Geometry check sheet. Reference: the model listing, model coordinates, mm. Face numbers are marked on the shaded views. A direction names the side the tool comes from. Coordinates: 2 decimals unless noted, no trailing zeros. Order: outer loops, then holes, each group sorted by start corner. A loop starts at its lowest first (then second) coordinate and runs counter-clockwise, first axis right, second up. Notation, with made-up numbers: M 88,-29.75 L 124,-29.75 A25 cw 124,-12.75 Z; hole C -5.75,82 d10. An arc over 180 degrees is marked long. Use CSV: the item, a comma, the result in double quotes. Start each with the question number.
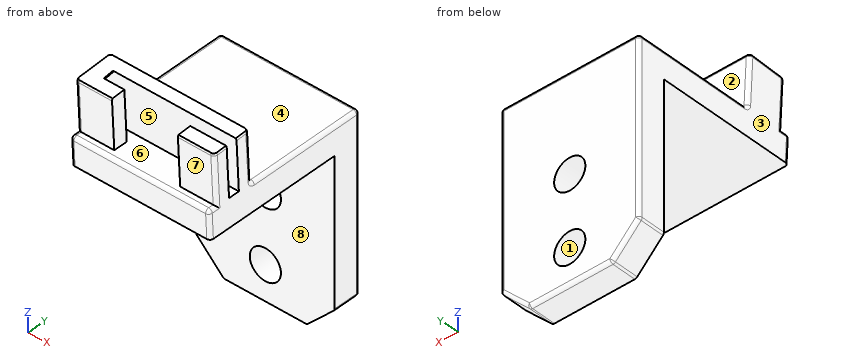
```python
from build123d import *

# Parameters (mm, degrees)
SKETCH1_W                       = 25.4
SKETCH1_H                       = 31.75
SKETCH1_R                       = 2.8575
BOSS_EXTRUDE1_DEPTH             = 5.08
BOSS_EXTRUDE2_REACH             = 22.955
BOSS_EXTRUDE2_DIRECTION_2_REACH = 22.955
CUT_EXTRUDE3_REACH              = 56.752
BOSS_EXTRUDE3_DEPTH             = 2
BOSS_EXTRUDE3_DRAFT             = -3
CHAMFER1_SIZE                   = 5.08
FILLET1_R                       = 0.635
SKETCH8_W                       = 25.4
SKETCH8_H                       = 6.35
CUT_EXTRUDE4_DEPTH              = 41.010145227


with BuildPart() as part:
    # Sketch1 → Boss-Extrude1 (new body)
    with BuildSketch(Plane(origin=(0, 0, 0), x_dir=(1, 0, 0), z_dir=(0, 1, 0))):
        Rectangle(SKETCH1_W, SKETCH1_H)
        with Locations(Location((0, 9.525, 0), (0, 0, 270))):
            Circle(SKETCH1_R, mode=Mode.SUBTRACT)
        with Locations(Location((0, -3.175, 0), (0, 0, 270))):
            Circle(SKETCH1_R, mode=Mode.SUBTRACT)
    extrude(amount=BOSS_EXTRUDE1_DEPTH)

    # Boss-Extrude2: up to this face of the body (flat: up to its plane)
    boss_extrude2_end = Plane(part.part.faces().sort_by_distance((12.7, 2.54, 0))[0])
    # Sketch2 → Boss-Extrude2 (add, up to the picked face)
    with BuildSketch(Plane(origin=(0, 0, 0), x_dir=(0, 0, -1), z_dir=(1, 0, 0)), mode=Mode.PRIVATE) as boss_extrude2_sk1:
        Polygon((-15.875, 5.08), (-20.955, 5.08), (-20.955, -17.014374457), (-30.831377514, -17.53197347), (-30.460838941, -24.60227064), (-21.059671916, -24.109576354), (-21.059671916, -25.671717141), (-15.875, -25.4), align=None)
    boss_extrude2_tool1 = split(extrude(boss_extrude2_sk1.sketch, amount=BOSS_EXTRUDE2_REACH, mode=Mode.PRIVATE), bisect_by=boss_extrude2_end, keep=Keep.BOTH, mode=Mode.PRIVATE)
    # Sketch2 → Boss-Extrude2 (add, up to the picked face)
    with BuildSketch(Plane(origin=(0, 0, 0), x_dir=(0, 0, -1), z_dir=(1, 0, 0)), mode=Mode.PRIVATE) as boss_extrude2_sk2:
        Polygon((-30.698444185, -20.068492489), (-30.593772269, -22.065751622), (-21.059671916, -21.566090595), (-21.059671916, -19.563345839), align=None)
    boss_extrude2_tool2 = split(extrude(boss_extrude2_sk2.sketch, amount=BOSS_EXTRUDE2_REACH, mode=Mode.PRIVATE), bisect_by=boss_extrude2_end, keep=Keep.BOTH, mode=Mode.PRIVATE)
    add(boss_extrude2_tool1.solids().sort_by(Axis((0, -13.472044, 20.681092), (1, 0, 0)))[0])
    add(boss_extrude2_tool2.solids().sort_by(Axis((0, -20.8141, 25.852938), (1, 0, 0)))[0])

    # Boss-Extrude2 direction 2: up to this face of the body (flat: up to its plane)
    boss_extrude2_direction_2_end = Plane(part.part.faces().sort_by_distance((-12.7, 2.54, 0))[0])
    # Sketch2 → Boss-Extrude2 direction 2 (add, up to the picked face)
    with BuildSketch(Plane(origin=(0, 0, 0), x_dir=(0, 0, -1), z_dir=(1, 0, 0)), mode=Mode.PRIVATE) as boss_extrude2_direction_2_sk1:
        Polygon((-15.875, 5.08), (-20.955, 5.08), (-20.955, -17.014374457), (-30.831377514, -17.53197347), (-30.460838941, -24.60227064), (-21.059671916, -24.109576354), (-21.059671916, -25.671717141), (-15.875, -25.4), align=None)
    boss_extrude2_direction_2_tool1 = split(extrude(boss_extrude2_direction_2_sk1.sketch, amount=-BOSS_EXTRUDE2_DIRECTION_2_REACH, mode=Mode.PRIVATE), bisect_by=boss_extrude2_direction_2_end, keep=Keep.BOTH, mode=Mode.PRIVATE)
    # Sketch2 → Boss-Extrude2 direction 2 (add, up to the picked face)
    with BuildSketch(Plane(origin=(0, 0, 0), x_dir=(0, 0, -1), z_dir=(1, 0, 0)), mode=Mode.PRIVATE) as boss_extrude2_direction_2_sk2:
        Polygon((-30.698444185, -20.068492489), (-30.593772269, -22.065751622), (-21.059671916, -21.566090595), (-21.059671916, -19.563345839), align=None)
    boss_extrude2_direction_2_tool2 = split(extrude(boss_extrude2_direction_2_sk2.sketch, amount=-BOSS_EXTRUDE2_DIRECTION_2_REACH, mode=Mode.PRIVATE), bisect_by=boss_extrude2_direction_2_end, keep=Keep.BOTH, mode=Mode.PRIVATE)
    add(boss_extrude2_direction_2_tool1.solids().sort_by(Axis((0, -13.472044, 20.681092), (-1, 0, 0)))[0])
    add(boss_extrude2_direction_2_tool2.solids().sort_by(Axis((0, -20.8141, 25.852938), (-1, 0, 0)))[0])

    # Cut-Extrude3: up to this plane
    cut_extrude3_end = Plane(origin=(46.895925715, 0, 21.059671916), z_dir=(0, 0, -1))
    # Sketch4 → Cut-Extrude3 (cut, up to the surface)
    with BuildSketch(Plane(origin=(0, -1.659399249, 31.663223881), x_dir=(1, 0, 0), z_dir=(0, -0.052335956242941094, 0.9986295347545742)), mode=Mode.PRIVATE) as cut_extrude3_sk1:
        Polygon((-11.43, -20.434356949), (-6.0325, -20.434356949), (-6.0325, -22.974356949), (6.0325, -22.974356949), (6.0325, -20.434356949), (12.7, -20.434356949), (12.7, -18.434356885), (-11.43, -18.434356885), align=None)
    cut_extrude3_tool1 = split(extrude(cut_extrude3_sk1.sketch, amount=-CUT_EXTRUDE3_REACH, mode=Mode.PRIVATE), bisect_by=cut_extrude3_end, keep=Keep.BOTH, mode=Mode.PRIVATE)
    add(cut_extrude3_tool1.solids().sort_by_distance((0.388379, -21.947535, 30.599968))[0], mode=Mode.SUBTRACT)


with BuildPart() as boss_extrude3_tool:
    # Sketch5 → Boss-Extrude3 (with draft: the straight prism first)
    with BuildSketch(Plane(origin=(0, -18.40909324, -0.964779695), x_dir=(1, 0, 0), z_dir=(0, -0.9986295347545742, -0.052335956242941115))):
        Polygon((-11.43, 29.674676779), (-9.906, 31.198676779), (-9.906, 31.706676779), (-11.43, 31.706676779), align=None)
    extrude(amount=BOSS_EXTRUDE3_DEPTH)
    # Boss-Extrude3: the draft: its side faces are tilted about the plane it starts from
    boss_extrude3_sides = [boss_extrude3_tool.faces().sort_by_distance(p)[0] for p in [
        (-10.668, -21.000655359, 29.37784872),
        (-9.906, -21.05382869, 30.392456327),
        (-10.668, -21.067122023, 30.646108229),
        (-11.43, -21.013948692, 29.631500622),
    ]]
    draft(boss_extrude3_sides, Plane(origin=(0, -18.40909324, -0.964779695), x_dir=(1, 0, 0), z_dir=(0, -0.9986295347545742, -0.052335956242941115)), BOSS_EXTRUDE3_DRAFT)


with BuildPart() as part_1:
    add(part.part)

    # Boss-Extrude3: add boss_extrude3_tool
    add(boss_extrude3_tool.part)

    # Chamfer1
    chamfer1_edges = [part_1.edges().sort_by_distance(p)[0] for p in [
        (-12.7, 2.54, -15.875),
        (12.7, 2.54, -15.875),
    ]]
    chamfer(chamfer1_edges, length=CHAMFER1_SIZE)

    # Fillet1
    fillet1_edges = [part_1.edges().sort_by_distance(p)[0] for p in [
        (12.7, -5.967187229, 20.955),
        (0, 5.08, 20.955),
        (12.7, -25.535858571, 18.467335958),
        (0, -25.671717141, 21.059671916),
        (12.7, -24.890646748, 21.059671916),
        (12.7, -24.355923497, 25.760255428),
        (9.36625, -24.60227064, 30.460838941),
        (12.7, -23.334011131, 30.527305605),
        (0, -17.53197347, 30.831377514),
        (12.7, -17.273173964, 25.893188757),
        (0, -17.014374457, 20.955),
        (-12.7, -17.273173964, 25.893188757),
        (-12.7, -5.967187229, 20.955),
        (-12.7, -25.535858571, 18.467335958),
        (-12.7, -24.890646748, 21.059671916),
        (-12.7, -24.355923497, 25.760255428),
        (-12.7, -21.067122055, 30.646108227),
        (-9.36625, -24.60227064, 30.460838941),
        (12.7, -18.800232979, 30.76491085),
        (12.7, 5.08, 5.08),
        (-12.7, 5.08, 5.08),
        (-12.7, 2.54, -10.795),
        (0, 5.08, -15.875),
        (7.62, 2.54, -15.875),
        (-7.62, 2.54, -15.875),
        (10.16, 5.08, -13.335),
        (-10.16, 5.08, -13.335),
        (12.7, 2.54, -10.795),
    ]]
    fillet(fillet1_edges, radius=FILLET1_R)

    # Sketch8 → Cut-Extrude4 (cut, through all)
    with BuildSketch(Plane(origin=(0, -15.872574222, -0.831846366), x_dir=(1, 0, 0), z_dir=(0, 0.9986295347545742, 0.05233595624294136))):
        with Locations((0, -34.627676779)):
            Rectangle(SKETCH8_W, SKETCH8_H)
    extrude(amount=-CUT_EXTRUDE4_DEPTH, mode=Mode.SUBTRACT)


solid = part_1.part
```
1) Material ranges on line 1 along Z through (x, y) = (1.25, -14) (3 decimals); line 2 along Y through (x, z) = (5.75, 4.5); line 3 along Y through (x, z) = (11.25, 24), recorded low to high.
2) Section check A-A on x = 0. Record the boundary of the cut face in (y, z) (1 decimal).
3) Section check B-B on x = 3.5. Record the boundary of the cut face in (y, z) (1 decimal).
4) Section check D-D on z = 14.5. Record the boundary of the cut face in (x, y) (3 decimals).
5) Draft check along X on the marked faces 1, 2 and 3. Enter one of: +X half, -X half, draft (parallel to the pull), parting line (faces both ways), or undercut.
6) Set-up check for the marked faces 4, 5, 6, 7 and 8: record each of +Z, -Z, +X, -X, +Y, -Y from which the full face is reachable in a straight line by a thin tool's end or side.
7) Gauge pin test, flat ends, axial feed: P1, Ø3, axis at x = -0.5, z = 23.5, coming from the -Y side; P2, Ø1, axis at x = -2.5, z = 24, coming from the -Y side; P3, Ø7.5, axis at x = -4.5, y = -6.5, coming from the -Z side (3 decimals); P4, Ø9, axis at x = 0, z = 3.175, coming from the +Y side. Record the tip position at first contact, or that the pin passes through.
8) Section check C-C on y = -4.5. Record the boundary of the cut face in (x, z) (3 decimals), then the cut area to 3 significant figures.
Results are:
1,line 1,"z = 15.875 to 20.955"
1,line 2,"y = 0 to 5.08"
1,line 3,"y = -24.26 to -21.72, -19.72 to -17.17"
2,outline,"M -25.6,20.4 L -25.4,15.9 L 0,15.9 L 0,6 L 5.1,6 L 5.1,20.3 A0.6 ccw 4.4,21 L -16.4,21 A0.6 cw -17,21.6 L -17.5,30.2 A0.6 ccw -17.6,30.6 L -20.1,30.4 L -19.6,21.1 L -25,21.1 A0.6 ccw Z; M 0,-15.9 L 4.4,-15.9 A0.6 ccw 5.1,-15.2 L 5.1,-12.4 L 0,-12.4 Z; M 0,-6.7 L 5.1,-6.7 L 5.1,0.3 L 0,0.3 Z"
3,outline,"M -25.6,20.4 L -25.4,15.9 L 0,15.9 L 0,-15.9 L 4.4,-15.9 A0.6 ccw 5.1,-15.2 L 5.1,20.3 A0.6 ccw 4.4,21 L -16.4,21 A0.6 cw -17,21.6 L -17.5,30.2 A0.6 ccw -17.6,30.6 L -20.1,30.4 L -19.6,21.1 L -25,21.1 A0.6 ccw Z"
4,outline,"M -12.7,0 L 12.7,0 L 12.7,4.445 A0.635 ccw 12.065,5.08 L -12.065,5.08 A0.635 ccw -12.7,4.445 Z"
5,face 1,"undercut"
5,face 2,"draft"
5,face 3,"-X half"
6,face 4,"+Z, +X, -X, +Y"
6,face 5,"+X"
6,face 6,"none"
6,face 7,"+X, -X, -Y"
6,face 8,"-Z, +X, -X, -Y"
7,P1,"stops at y = -19.77"
7,P2,"stops at y = -19.74"
7,P3,"stops at z = 15.875"
7,P4,"stops at y = 5.08"
8,outline,"M -12.7,15.875 L 12.7,15.875 L 12.7,20.32 A0.635 ccw 12.065,20.955 L -12.065,20.955 A0.635 ccw -12.7,20.32 Z"
8,area,"129 mm²"
